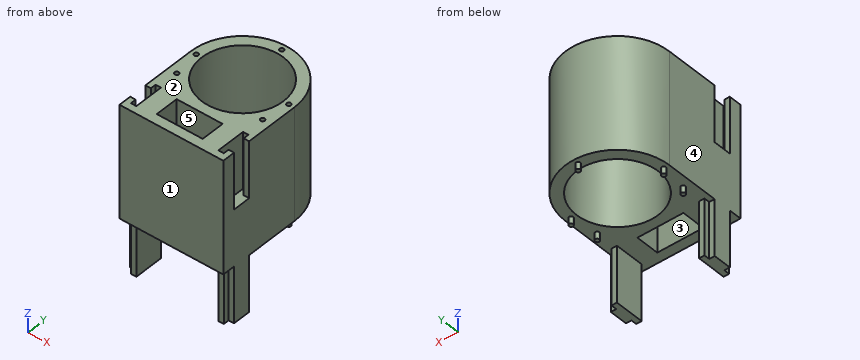
```python
from build123d import *

# Parameters (mm, degrees)
F0_W      = 41.476287
F0_H      = 21.196319
F0_R      = 36.83
F1_DEPTH  = 101.6
F4_DEPTH  = 50.8
F6_DEPTH  = 50.8
F7_R      = 1.918424
F7_R_2    = 1.918426
F8_DEPTH  = 6.35
F9_R      = 1.918426
F10_DEPTH = 6.35


with BuildPart() as f1:
    # F0 (on Top) → F1 (new body)
    with BuildSketch(Plane.XY):
        with BuildLine():
            Line((61.68938, -26.920194), (61.68938, 48.886125))
            ThreePointArc((61.68938, 48.886125), (14.852995, 95.72251), (-31.98339, 48.886125))
            Line((-31.98339, 48.886125), (-31.98339, -26.920194))
            Line((-31.98339, -26.920194), (61.68938, -26.920194))
        make_face()
        with Locations((14.852995, -7.432034)):
            Rectangle(F0_W, F0_H, mode=Mode.SUBTRACT)
        with Locations((14.852995, 48.886125)):
            Circle(F0_R, mode=Mode.SUBTRACT)
    extrude(amount=F1_DEPTH)

    # F3 (on face) → F4 (join)
    with BuildSketch(Plane(origin=(0, 0, 0), x_dir=(1, 0, 0), z_dir=(0, 0, -1))):
        Polygon((51.882841, 20.570194), (51.882841, 20.069338), (51.882841, -5.706131), (56.786107, -5.706131), (56.786107, -0.626131), (61.68938, -0.626131), (61.68938, 15.490194), (56.78611, 15.490194), (56.78611, 20.069338), (56.78611, 20.570194), align=None)
        Polygon((-22.17685, -5.706131), (-22.17685, 20.069338), (-22.17685, 20.570194), (-27.08012, 20.570194), (-27.08012, 20.069338), (-27.08012, 15.490194), (-31.98339, 15.490194), (-31.98339, -0.626131), (-27.080117, -0.626131), (-27.080117, -5.706131), align=None)
    extrude(amount=F4_DEPTH)

    # F5 (on face) → F6 (cut)
    with BuildSketch(Plane.XY.offset(101.6)):
        Polygon((-31.98339, 0.626131), (-31.98339, -15.490194), (-27.080123, -15.490194), (-27.080123, -20.570194), (-22.176856, -20.570194), (-22.176856, -15.490194), (-22.176856, 0.626131), (-22.176856, 5.706131), (-27.080123, 5.706131), (-27.080123, 0.626131), align=None)
        Polygon((51.882846, 0.626131), (51.882846, -15.490194), (51.882846, -20.570194), (56.786113, -20.570194), (56.786113, -15.490194), (61.68938, -15.490194), (61.68938, 0.626131), (56.786113, 0.626131), (56.786113, 5.706131), (51.882846, 5.706131), align=None)
    extrude(amount=-F6_DEPTH, mode=Mode.SUBTRACT)

    # F7 (on face) → F8 (cut)
    with BuildSketch(Plane.XY.offset(101.6)):
        with Locations((-26.980197, 48.886125)):
            Circle(F7_R)
        with Locations((-23.892931, 24.574445)):
            Circle(F7_R)
        with Locations((53.598921, 24.574445)):
            Circle(F7_R)
        with Locations((56.686187, 48.886125)):
            Circle(F7_R)
        with Locations((14.852995, 90.719925)):
            Circle(F7_R_2)
    extrude(amount=-F8_DEPTH, mode=Mode.SUBTRACT)

    # F9 (on face) → F10 (join)
    with BuildSketch(Plane(origin=(0, 0, 0), x_dir=(1, 0, 0), z_dir=(0, 0, -1))):
        with Locations((56.686187, -48.886125)):
            Circle(F9_R)
        with Locations((14.852995, -90.719925)):
            Circle(F9_R)
        with Locations((-26.980197, -48.886125)):
            Circle(F9_R)
        with Locations((-23.892931, -24.574445)):
            Circle(F9_R)
        with Locations((53.598921, -24.574445)):
            Circle(F9_R)
    extrude(amount=F10_DEPTH)


solid = f1.part
```
Check sheet for the modelled part. Datum: model origin and axes. Units: mm. Face numbers are marked on the shaded views. A direction names the side the tool comes from. Coordinates: 2 decimals unless noted, no trailing zeros. Order: outer loops, then holes, each group sorted by start corner. A loop starts at its lowest first (then second) coordinate and runs counter-clockwise, first axis right, second up. Notation, with made-up numbers: M -30,19.25 L 8,19.25 A13 cw 8,23.25 Z; hole C 70,50 d9. An arc over 180 degrees is marked long. Write each question's results on one line, items separated by ' | '. Start each with the question number.
1. Mould release check, pull along Y, two halves, no side actions. Record for the marked faces 1, 2 and 3: +Y half, -Y half, draft (parallel to the pull), parting line (faces both ways), or undercut.
2. Access from +Z, -Z, +X, -X, +Y, -Y to the whole of each face (thin tool, end or side, straight path). Record for the marked faces 4 and 5.
3. Cross-section at C-C on x = -8. Record the cut outline in (y, z), and give its area (3 significant figures).
4. Go/stop test with flat-tipped pins: P1, Ø6, axis at x = 45, y = 59, coming from the +Z side; P2, Ø4, axis at y = 72.5, z = 73, coming from the -X side; P3, Ø3, axis at x = 14, y = 91, coming from the -Z side; P4, Ø4, axis at x = 60.5, z = -24, coming from the -Y side. Record where each tip stops, or that it passes through.
5. Material ranges on probe 1 along Y at (x, z) = (4.5, 44); probe 2 along X at (y, z) = (-8, -29); probe 3 along X at (y, z) = (-15, 38), recorded low to high.
6. Cross-section at D-D on x = 29. Record the cut outline in (y, z), and give its area (3 significant figures).
7. Cross-section at A-A on y = -7.5. Record the cut outline in (x, z), and give its area (3 significant figures).
Checks:
1) face 1: -Y half | face 2: draft | face 3: undercut
2) face 4: +Z, -Z, -X, +Y, -Y | face 5: +Z, -Z
3) outline: M -26.92,0 L 20,0 L 20,101.6 L -26.92,101.6 Z; M 77.77,0 L 89.77,0 L 89.77,101.6 L 77.77,101.6 Z | area: 5,990 mm²
4) P1: passes through | P2: stops at x = -26.7 | P3: stops at z = -6.35 | P4: stops at y = -15.49
5) probe 1: y = -26.92 to -18.03, 3.17 to 13.54, 84.23 to 94.56 | probe 2: x = -31.98 to -22.18, 51.88 to 61.69 | probe 3: x = -31.98 to -5.89, 35.59 to 61.69
6) outline: M -26.92,0 L -18.03,0 L -18.03,101.6 L -26.92,101.6 Z; M 3.17,0 L 14.88,0 L 14.88,101.6 L 3.17,101.6 Z; M 82.89,0 L 93.53,0 L 93.53,101.6 L 82.89,101.6 Z | area: 3,170 mm²
7) outline: M -31.98,-50.8 L -22.18,-50.8 L -22.18,0 L -5.89,0 L -5.89,101.6 L -22.18,101.6 L -22.18,50.8 L -31.98,50.8 Z; M 35.59,0 L 51.88,0 L 51.88,-50.8 L 61.69,-50.8 L 61.69,50.8 L 51.88,50.8 L 51.88,101.6 L 35.59,101.6 Z | area: 5,300 mm²
